Read the model definition and answer for the solid it produces. Units are mm, in the model's axes. A direction names the side the tool comes from. Coordinates: 2 decimals unless noted, no trailing zeros. Write each loop counter-clockwise with the first axis right and the second up, starting at its lowest first coordinate (ties: lowest second). Pieces come first, ordered by that corner, then holes.
from build123d import *

# Parameters (mm, degrees)
F0_W     = 83.6216490716
F0_H     = 83.1985995173
F1_DEPTH = 40
F2_W     = 41.8108245358
F2_H     = 83.1985995173
F3_DEPTH = 40
F4_R     = 5


with BuildPart() as f1:
    # F0 (on Top) → F1 (new body)
    with BuildSketch(Plane.XY):
        with Locations((-17.3164242879, -4.335001111)):
            Rectangle(F0_W, F0_H)
    extrude(amount=F1_DEPTH)

    # F2 (on face) → F3 (join)
    with BuildSketch(Plane.XY.offset(40)):
        with Locations((-38.2218365557, -4.335001111)):
            Rectangle(F2_W, F2_H)
    extrude(amount=F3_DEPTH)

    # F4
    f4_edges = [f1.edges().sort_by_distance(p)[0] for p in [
        (-17.316424, -4.335001, 40),
        (-59.127249, 37.264299, 40),
        (-59.127249, -4.335001, 80),
        (-59.127249, -45.934301, 40),
        (-59.127249, -4.335001, 0),
        (3.588988, 37.264299, 40),
        (3.588988, -45.934301, 40),
        (24.4944, 37.264299, 20),
        (-17.316424, 37.264299, 60),
        (-38.221837, 37.264299, 80),
        (-17.316424, 37.264299, 0),
        (-17.316424, -45.934301, 60),
        (-17.316424, -45.934301, 0),
        (24.4944, -4.335001, 0),
        (24.4944, -4.335001, 40),
        (-17.316424, -4.335001, 80),
        (-38.221837, -45.934301, 80),
        (24.4944, -45.934301, 20),
    ]]
    fillet(f4_edges, radius=F4_R)


solid = f1.part
Item 1: The part is cut by section A-A (z = 65). Give the vertices of the cut face in (x, y), and give its area (3 significant figures).
Item 2: For faces 1 (the cylindrical face through (3.812, 35.838, 38.496)), 2 (the cylindrical face through (3.812, -44.508, 38.496)), 3 (the cylindrical face through (-16.801, 35.838, 1.504)), determine the directions among +Z, -Z, +X, -X, +Y, -Y from which every point of the face is accessible in a straight line to the end or side of a thin tool.
Item 3: Find the intervals of material crossed by probe 1 along Z at (x, y) = (18, 1); probe 2 along X at (y, z) = (21, 50); probe 3 along Y at (x, z) = (-54.5, 53), in increasing order.
Item 4: The part is cut by section B-B (x = 5.5). Give the vertices of the cut face in (y, z).
Item 5: The part is cut by section C-C (y = -11). Give the vertices of the cut face in (x, z).
Item 6: Given pin 1 (6 mm diameter, centred on x = 1, y = -15.5, fed in from +Z); pin 2 (3 mm diameter, centred on y = 13.5, z = 72, fed in from +X), each flat-ended and moving along its own axis, determine where each tip first touches the part or whether it passes through.
Answer:
1. outline: (-59.13, -40.93) arc R5 ccw to (-54.13, -45.93) - (-22.32, -45.93) arc R5 ccw to (-17.32, -40.93) - (-17.32, 32.26) arc R5 ccw to (-22.32, 37.26) - (-54.13, 37.26) arc R5 ccw to (-59.13, 32.26) - close
1. area: 3,460 mm2
2. face 1: +Z, +X, +Y
2. face 2: +Z, +X, -Y
2. face 3: -Z, +X, -X, +Y
3. probe 1: z = 0 to 40
3. probe 2: x = -59.13 to -17.32
3. probe 3: y = -45.92 to 37.25
4. outline: (-45.93, 5) arc R5 ccw to (-40.93, 0) - (32.26, 0) arc R5 ccw to (37.26, 5) - (37.26, 35) arc R5 ccw to (32.26, 40) - (-40.93, 40) arc R5 ccw to (-45.93, 35) - close
5. outline: (-59.13, 5) arc R5 ccw to (-54.13, 0) - (19.49, 0) arc R5 ccw to (24.49, 5) - (24.49, 35) arc R5 ccw to (19.49, 40) - (-12.32, 40) arc R5 cw to (-17.32, 45) - (-17.32, 75) arc R5 ccw to (-22.32, 80) - (-54.13, 80) arc R5 ccw to (-59.13, 75) - close
6. pin 1: stops at z = 40
6. pin 2: stops at x = -17.32
